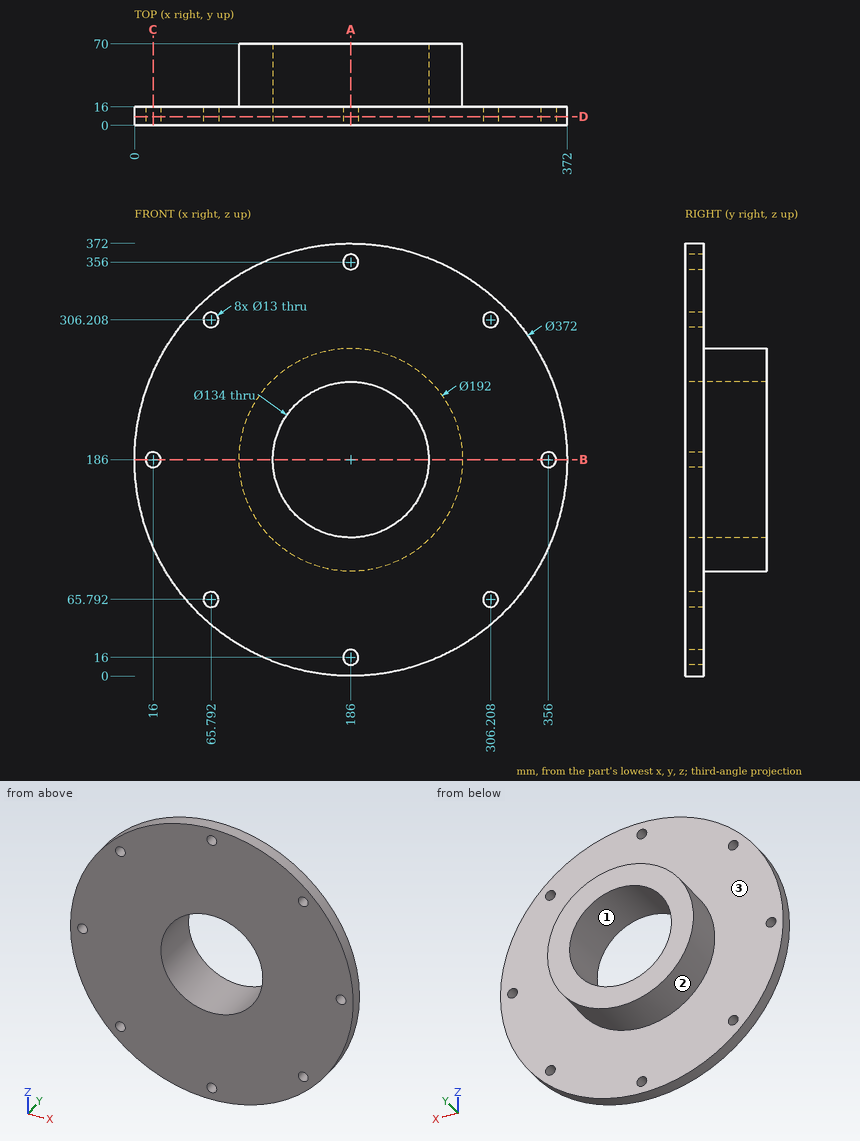
Input: dimensioned drawing with shaded views. Units: mm. Origin: part minimum x, y, z. Coordinates: 2 decimals unless noted, no trailing zeros. Loops run counter-clockwise (first coordinate to the right, second up) from the corner with the lowest first, then second, coordinate; pieces in that order, holes last. Notation, with made-up numbers: (50, -21.75) -> (99, -21.75) arc R29 cw to (99, -0.75) -> close; hole circle Ø7 at (72.5, 61.5). An arc over 180 degrees is marked (long way). Use a Markdown table: item, result. Add a question column.
(1) Section query A-A, the plane x = 186. Return loops of the section in (y, z), plus the area to 3 significant figures.
(2) Section query C-C, the plane x = 16. Return loops of the section in (y, z), plus the area to 3 significant figures.
(3) Mould query, pull axis Z, two halves, no side actions, for the marked faces 1, 2 and 3. Classes: pulls with the +Z half, pulls with the -Z half, needs draft (parallel to the pull), parting line crosses it, or undercut.
(4) Section query D-D, the plane y = 7.5. State how many separate pieces and enclosed holes the cut face has, plus the area to 3 significant figures.
(5) Line query: line 1 along X through (y, z) = (10, 71); line 2 along Z through (x, y) = (184.5, 37); line 3 along Y through (x, z) = (224, 354). Output: solid intervals per line, ascending.
(6) Section query B-B, the plane z = 186. Return loops of the section in (x, y).
(7) Pin query (flat end, axial travel): pin 1 Ø6 at (y, z) = (51, 167.5) entering from -X; pin 2 Ø4 at (x, y) = (259, 25) entering from -Z; pin 3 Ø6 at (y, z) = (34.5, 244) entering from +X. Return the tip coordinate at first contact, or that it passes through.
Answer:
| question | item | result |
|---|---|---|
| 1 | outline | (0, 0) -> (16, 0) -> (16, 9.5) -> (0, 9.5) -> close; (0, 22.5) -> (16, 22.5) -> (16, 90) -> (70, 90) -> (70, 119) -> (0, 119) -> close; (0, 253) -> (70, 253) -> (70, 282) -> (16, 282) -> (16, 349.5) -> (0, 349.5) -> close; (0, 362.5) -> (16, 362.5) -> (16, 372) -> (0, 372) -> close |
| 1 | area | 6,520 mm^2 |
| 2 | outline | (0, 110.53) -> (16, 110.53) -> (16, 179.5) -> (0, 179.5) -> close; (0, 192.5) -> (16, 192.5) -> (16, 261.47) -> (0, 261.47) -> close |
| 2 | area | 2,210 mm^2 |
| 3 | face 1 | undercut |
| 3 | face 2 | parting line crosses it |
| 3 | face 3 | needs draft |
| 4 | separate pieces | 1 |
| 4 | enclosed holes | 9 |
| 4 | area | 93,500 mm^2 |
| 5 | line 1 | x = 39.81 to 61.9, 69.68 to 302.32, 310.1 to 332.19 |
| 5 | line 2 | z = 90.01 to 119.02, 252.98 to 281.99 |
| 5 | line 3 | y = 0 to 16 |
| 6 | outline | (0, 0) -> (9.5, 0) -> (9.5, 16) -> (0, 16) -> close; (22.5, 0) -> (119, 0) -> (119, 70) -> (90, 70) -> (90, 16) -> (22.5, 16) -> close; (253, 0) -> (349.5, 0) -> (349.5, 16) -> (282, 16) -> (282, 70) -> (253, 70) -> close; (362.5, 0) -> (372, 0) -> (372, 16) -> (362.5, 16) -> close |
| 7 | pin 1 | stops at x = 91.26 |
| 7 | pin 2 | stops at z = 121.39 |
| 7 | pin 3 | stops at x = 264.68 |
